```python
from build123d import *

# Parameters (mm, degrees)
F0_W     = 101.6
F0_H     = 50.8
F1_DEPTH = 25.4
F3_D     = 6.5278
F4_R     = 5.08
F5_R     = 5.08
F6_R     = 5.08


with BuildPart() as f1:
    # F0 (on Top) → F1 (new body)
    with BuildSketch(Plane.XY):
        with Locations((50.8, 25.4)):
            Rectangle(F0_W, F0_H)
    extrude(amount=F1_DEPTH)

    # F3 (through all)
    with Locations(Plane.XY.offset(25.4)):
        with Locations((67.2795102, 25.5870483816)):
            Hole(F3_D / 2)

    # F4
    f4_edges = [f1.edges().sort_by_distance(p)[0] for p in [
        (101.6, 50.8, 12.7),
        (101.6, 0, 12.7),
        (0, 0, 12.7),
        (0, 50.8, 12.7),
    ]]
    fillet(f4_edges, radius=F4_R)

    # F5
    f5_edges = [f1.edges().sort_by_distance(p)[0] for p in [
        (101.6, 25.4, 25.4),
    ]]
    fillet(f5_edges, radius=F5_R)

    # F6
    f6_edges = [f1.edges().sort_by_distance(p)[0] for p in [
        (101.6, 25.4, 0),
    ]]
    fillet(f6_edges, radius=F6_R)


solid = f1.part
```
Here's how the part is built. I have some questions about the finished solid (model axes, mm). Give positions to 0.01 mm unless a question says otherwise; leave off trailing zeros. Loops run counter-clockwise (first coordinate to the right, second up) from the corner with the lowest first, then second, coordinate; pieces in that order, holes last. Notation, with made-up numbers: (2, 45.5) -> (39, 45.5) arc R15 ccw to (39, 56.5) -> close; hole circle Ø4 at (68, 86). An arc over 180 degrees is marked (long way). Use one line per item in the form item = value. Start each with the question number.
1) Thinking about a two-plate mould opening in X: for faces 1 (the face through (50, 26, 0)), 2 (the face through (1.449, 1.528, 12.807)), 3 (the face through (69.69, 27.79, 12.52)), which applies, +X half, -X half, draft (parallel to the pull), parting line (faces both ways), or undercut?
2) Please list where these lines run through material, in increasing order: line 1 along Y through (x, z) = (13.5, 20.75); line 2 along Y through (x, z) = (13.5, 2.75); line 3 along X through (y, z) = (4, 8).
3) Imagine slicing it at B-B (z = 3.25). Please give me the cut outline in (x, y).
4) Imagine slicing it at D-D (y = 3.5). Please give me the cut outline in (x, z).
5) Imagine slicing it at A-A (x = 58.5). Please give me the cut outline in (y, z).
6) Imagine slicing it at C-C (y = 27.5). Please give me the cut outline in (x, z).
Check values:
q1.face_1 = draft
q1.face_2 = -X half
q1.face_3 = undercut
q2.line_1 = 0.02 to 50.78
q2.line_2 = 0.57 to 50.23
q2.line_3 = 0.12 to 101.48
q3.outline = (0.34, 5.08) arc R4.74 ccw to (5.08, 0.34) -> (96.52, 0.34) arc R4.74 ccw to (101.26, 5.08) -> (101.26, 45.72) arc R4.74 ccw to (96.52, 50.46) -> (5.08, 50.46) arc R4.74 ccw to (0.34, 45.72) -> close; hole circle Ø6.53 at (67.28, 25.59)
q4.outline = (0.25, 5.08) arc R4.83 ccw to (5.08, 0.25) -> (96.52, 0.25) arc R4.83 ccw to (101.35, 5.08) -> (101.35, 20.32) arc R4.83 ccw to (96.52, 25.15) -> (5.08, 25.15) arc R4.83 ccw to (0.25, 20.32) -> close
q5.outline = (0, 5.08) arc R5.08 ccw to (5.08, 0) -> (45.72, 0) arc R5.08 ccw to (50.8, 5.08) -> (50.8, 20.32) arc R5.08 ccw to (45.72, 25.4) -> (5.08, 25.4) arc R5.08 ccw to (0, 20.32) -> close
q6.outline = (0, 5.08) arc R5.08 ccw to (5.08, 0) -> (64.63, 0) -> (64.63, 25.4) -> (5.08, 25.4) arc R5.08 ccw to (0, 20.32) -> close; (69.92, 0) -> (96.52, 0) arc R5.08 ccw to (101.6, 5.08) -> (101.6, 20.32) arc R5.08 ccw to (96.52, 25.4) -> (69.92, 25.4) -> close
